Design review of the part built by this model. Coordinates are the model's own, in mm. Coordinates: 2 decimals unless noted, no trailing zeros. Write each loop counter-clockwise with the first axis right and the second up, starting at its lowest first coordinate (ties: lowest second). Pieces come first, ordered by that corner, then holes. Notation, with made-up numbers: (50.25, 59) -> (74.25, 59) arc R16 cw to (74.25, 63) -> close; hole circle Ø3 at (21, -32). An arc over 180 degrees is marked (long way). Return JSON: item names as keys, results as strings. Group by question number.
Autodesk Inventor part; units mm, degrees
ref_plane "YZ Plane" through (0, 0, 0) normal (1, 0, 0) x (0, 1, 0)
ref_plane "XZ Plane" through (0, 0, 0) normal (0, 1, 0) x (-1, 0, 0)
ref_plane "XY Plane" through (0, 0, 0) normal (0, 0, 1) x (1, 0, 0)
sketch "Sketch1" plane through (0, 0, 0) normal (0, 1, 0) x (-1, 0, 0)
  circle A0 centre (0, 0) radius 70
  dimension "d0" = 140
extrude "Extrusion1" add sketch "Sketch1" along normal blind 1
sketch "Sketch2" plane through (0, 0, 0) normal (0, -1, 0) x (1, 0, 0)
  line L0 (0, 0) -> (36.3053, 37.4305)
  line L1 (36.3053, 37.4305) -> (28.3938, 45.1042)
  line L2 (28.3938, 45.1042) -> (20.7201, 37.1927)
  line L3 (20.7201, 37.1927) -> (28.6316, 29.519)
  line L4 (36.5432, 21.8453) -> (44.2169, 29.7568)
  line L5 (44.2169, 29.7568) -> (36.3053, 37.4305)
  line L6 (28.6316, 29.519) -> (36.5432, 21.8453)
extrude "Extrusion2" add sketch "Sketch2" along normal blind 10
sketch "Sketch3" plane through (28.3938, -10, 45.1042) normal (0.6962355, 0, 0.7178134) x (0.7178134, 0, -0.6962355)
  circle A0 centre (11.0217, 5.114) radius 2.5
  point P0 (11.0217, 10)
  dimension "d5" = 5
extrude "Extrusion3" add sketch "Sketch3" along normal blind 418.75
pattern_circular "Circular Pattern1" count 4 over 360 about axis through (0, 0, 0) along (0, 1, 0) of "Extrusion2", "Extrusion3"
properties part number "Spinning Platform"
Q1. The part is to be moulded in two halves that separate along X. For faces 1 (the cylindrical face through (55.55, 0.493, 42.594)), 2 (the flat face through (34, -10, -32)), 3 (the cylindrical face through (178.25, -5, 187.36)), say which applies: +X half, -X half, draft (parallel to the pull), parting line (faces both ways), or undercut.
Q2. We need section A-A on x = 0. Write out the cut boundary in (y, z), plus the area to 3 significant figures.
Q3. For P1, Ø1, axis at x = -29.5, y = -8, coming from the +Z side; P2, Ø1.5, axis at y = -7, z = 257, coming from the -X side; P3, Ø4, axis at y = -1.5, z = 35.5, coming from the -X side, all flat-tipped, find the tip position at first contact; note any pin that passes through.
Q4. Wall thickness on L1, parallel to Z at x = 210, y = -4.5; L2, parallel to X at y = -3.75, z = -249.5; L3, parallel to X at y = -3.75, z = 194.5: over which ranges is each line inside the solid? List them lowest first.
Q5. We need section B-B on z = 0. Write out the cut boundary in (x, y).
Findings below:
{
 "1": {"face 1": "parting line", "face 2": "draft", "face 3": "undercut"},
 "2": {"outline": "(0, -70) -> (1, -70) -> (1, 70) -> (0, 70) -> close", "area": "140 mm^2"},
 "3": {"P1": "stops at z = 44.22", "P2": "stops at x = -268.29", "P3": "stops at x = -61.09"},
 "4": {"L1": "z = -207.13 to -200.25, 212.96 to 220.06", "L2": "x = -245.1 to -238.9, 254.03 to 260.43", "L3": "x = -203.73 to -197.33, 185.55 to 191.76"},
 "5": {"outline": "(-70, 0) -> (70, 0) -> (70, 1) -> (-70, 1) -> close"}
}
